CAD build for the part. Positions are in the model's coordinates, mm. A direction names the side the tool comes from. Give positions to 0.01 mm unless a question says otherwise; leave off trailing zeros. Write each loop counter-clockwise with the first axis right and the second up, starting at its lowest first coordinate (ties: lowest second). Pieces come first, ordered by that corner, then holes. Notation, with made-up numbers: (81.25, 83) -> (118.25, 83) arc R17 cw to (118.25, 103) -> close; hole circle Ø9 at (-15.5, -16.5). An arc over 180 degrees is marked (long way). Use one line per item in the form item = value. Start each with the question number.
from build123d import *

# Parameters (mm, degrees)
EXTRUDE_THIN1_DEPTH     = 6.35
SKETCH4_R               = 2.286
CUT_EXTRUDE1_DEPTH      = 1
CUT_EXTRUDE1_DEPTH_BACK = 26.4
SKETCH5_R               = 2.286
CUT_EXTRUDE2_DEPTH      = 3.54


with BuildPart() as part:
    # Sketch1 → Extrude-Thin1 (new body, symmetric)
    with BuildSketch(Plane(origin=(0, 0, 0), x_dir=(0, 0, -1), z_dir=(1, 0, 0))):
        Polygon((-12.7, 25.4), (-12.7, 0), (12.7, 0), (12.7, 25.4), (10.16, 25.4), (10.16, 2.54), (-10.16, 2.54), (-10.16, 25.4), align=None)
    extrude(amount=EXTRUDE_THIN1_DEPTH, both=True)

    # Sketch4 → Cut-Extrude1 (cut, two sides)
    with BuildSketch(Plane.XY.offset(12.7)) as cut_extrude1_sk:
        with Locations((0, 21.1074)):
            Circle(SKETCH4_R)
    extrude(amount=CUT_EXTRUDE1_DEPTH, mode=Mode.SUBTRACT)
    extrude(cut_extrude1_sk.sketch, amount=-CUT_EXTRUDE1_DEPTH_BACK, mode=Mode.SUBTRACT)

    # Sketch5 → Cut-Extrude2 (cut, through all)
    with BuildSketch(Plane(origin=(0, 2.54, 0), x_dir=(1, 0, 0), z_dir=(0, 1, 0))):
        Circle(SKETCH5_R)
    extrude(amount=-CUT_EXTRUDE2_DEPTH, mode=Mode.SUBTRACT)


solid = part.part
1) Two-plate mould, pull along Z, no slides. Class faces 3 (the face through (0, 14, 10.16)), 4 (the face through (0, 0, -3)), 5 (the face through (0, 13, -12.7)), 6 (the face through (0, 14, -10.16)): released by +Z, released by -Z, zero draft, split by the parting line, or undercut.
2) Wall check: line 1 along Z through (x, y) = (-0.5, 8); line 2 along X through (y, z) = (0.75, 0); line 3 along Y through (x, z) = (0, -10.75). Give the ranges that are in metal, low to high. Write a range as from..to.
3) Cut at B-B (y = 15.5). Give the cut face in (x, z).
4) Pin check, flat tips, straight feed: pin 1 (5.5 mm diameter, centred on x = 0, z = 0, fed in from +Y); pin 2 (3.5 mm diameter, centred on x = 0, y = 21.11, fed in from -Z). Stop position of each tip, or through.
5) Cut at C-C (z = 0). Give the cut face in (x, y), and give its area (3 significant figures).
6) 3-axis set-ups, long thin cutter, end or side, ignore diameter. For faces 1 (the face through (-0.496, 18.876, -11.412)), 2 (the face through (-1.3, 2.54, -2.4)): which of +Z, -Z, +X, -X, +Y, -Y reach the whole face in a straight line?
7) Cut at A-A (x = 0). Give the cut face in (y, z), and give its area (3 significant figures).
8) Cut at D-D (x = -4.75). Give the cut face in (y, z).
Final values:
q1.face_3 = undercut
q1.face_4 = zero draft
q1.face_5 = released by -Z
q1.face_6 = undercut
q2.line_1 = -12.7..-10.16, 10.16..12.7
q2.line_2 = -6.35..-2.29, 2.29..6.35
q2.line_3 = 0..18.82, 23.39..25.4
q3.outline = (-6.35, -12.7) -> (6.35, -12.7) -> (6.35, -10.16) -> (-6.35, -10.16) -> close; (-6.35, 10.16) -> (6.35, 10.16) -> (6.35, 12.7) -> (-6.35, 12.7) -> close
q4.pin_1 = 2.54
q4.pin_2 = through
q5.outline = (-6.35, 0) -> (-2.29, 0) -> (-2.29, 2.54) -> (-6.35, 2.54) -> close; (2.29, 0) -> (6.35, 0) -> (6.35, 2.54) -> (2.29, 2.54) -> close
q5.area = 20.6 mm^2
q6.face_1 = +Z, -Z
q6.face_2 = +X, -X, +Y
q7.outline = (0, -12.7) -> (18.82, -12.7) -> (18.82, -10.16) -> (2.54, -10.16) -> (2.54, -2.29) -> (0, -2.29) -> close; (0, 2.29) -> (2.54, 2.29) -> (2.54, 10.16) -> (18.82, 10.16) -> (18.82, 12.7) -> (0, 12.7) -> close; (23.39, -12.7) -> (25.4, -12.7) -> (25.4, -10.16) -> (23.39, -10.16) -> close; (23.39, 10.16) -> (25.4, 10.16) -> (25.4, 12.7) -> (23.39, 12.7) -> close
q7.area = 146 mm^2
q8.outline = (0, -12.7) -> (25.4, -12.7) -> (25.4, -10.16) -> (2.54, -10.16) -> (2.54, 10.16) -> (25.4, 10.16) -> (25.4, 12.7) -> (0, 12.7) -> close
